Could you check a few things on this model? Use its own coordinates, in mm. Face numbers are marked on the shaded views. A direction names the side the tool comes from. Coordinates: 2 decimals unless noted, no trailing zeros. Order: outer loops, then holes, each group sorted by start corner. A loop starts at its lowest first (then second) coordinate and runs counter-clockwise, first axis right, second up. Notation, with made-up numbers: (22.5, 34.25) - (55.5, 34.25) arc R20 ccw to (55.5, 40.25) - close; hole circle Ø5 at (2, 56.25). An arc over 180 degrees is marked (long way). Answer as CSV lines item,"result". Start each with the question number.
1. I want a section at A-A, the plane z = 7. List the corners of the cut face in (x, y) for me.
2. Thinking about a two-plate mould opening in Y: for the marked faces 4, 5 and 6, which applies, released by +Y, released by -Y, zero draft, split by the parting line, or undercut?
3. For the marked faces 1, 2 and 3, which set-ups out of +Z, -Z, +X, -X, +Y, -Y let a thin tool reach every point of the face, with its end or its side?
4. I want a section at B-B, the plane y = 0. List the corners of the cut face in (x, z) for me (3 decimals).
5. For pin 1 (4 mm diameter, centred on x = 0.43, y = 0, fed in from -Z); pin 2 (3 mm diameter, centred on x = 0.5, y = -2.5, fed in from +Z) (3 decimals), each with a flat end and sliding along its axis, tell me the tip position at first contact or that it passes through.
6. I want a section at C-C, the plane x = 1.25. List the corners of the cut face in (y, z) for me (3 decimals), and give its area (3 significant figures).
7. I need wall thicknesses on probe 1 along Y at (x, z) = (0.5, 3.75); probe 2 along Y at (x, z) = (5.5, 4.25); probe 3 along X at (y, z) = (-1.25, 3). Which ranges of each line are inside material? Lowest first, please.
8. I want a section at D-D, the plane y = -3. List the corners of the cut face in (x, z) for me (3 decimals).
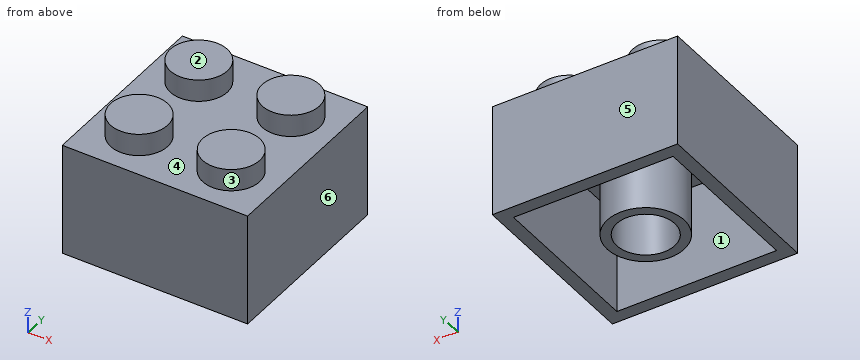
from build123d import *

# Parameters (mm, degrees)
F0_W     = 15.748
F0_H     = 15.748
F1_DEPTH = 9.525
F2_R     = 2.4257
F3_DEPTH = 1.8796
F4_W     = 13.5636
F4_H     = 13.5636
F5_DEPTH = 8.4328
F6_R     = 3.267
F7_DEPTH = 8.4328
F8_R     = 2.467
F9_DEPTH = 8.4328


with BuildPart() as f1:
    # F0 (on Top) → F1 (new body)
    with BuildSketch(Plane.XY):
        with Locations((0.432258, 0.097535)):
            Rectangle(F0_W, F0_H)
    extrude(amount=F1_DEPTH)

    # F2 (on face) → F3 (join)
    with BuildSketch(Plane.XY.offset(9.525)):
        with Locations((-3.479342, 4.009135)):
            Circle(F2_R)
        with Locations((4.343858, 4.009135)):
            Circle(F2_R)
        with Locations((-3.479342, -3.814065)):
            Circle(F2_R)
        with Locations((4.343858, -3.814065)):
            Circle(F2_R)
    extrude(amount=F3_DEPTH)

    # F4 (on face) → F5 (cut)
    with BuildSketch(Plane(origin=(0, 0, 0), x_dir=(1, 0, 0), z_dir=(0, 0, -1))):
        with Locations((0.432258, -0.097535)):
            Rectangle(F4_W, F4_H)
    extrude(amount=-F5_DEPTH, mode=Mode.SUBTRACT)

    # F6 (on face) → F7 (join)
    with BuildSketch(Plane(origin=(0, 0, 8.4328), x_dir=(1, 0, 0), z_dir=(0, 0, -1))):
        with Locations((0.431654, 0)):
            Circle(F6_R)
    extrude(amount=F7_DEPTH)

    # F8 (on face) → F9 (cut)
    with BuildSketch(Plane(origin=(0, 0, 0), x_dir=(1, 0, 0), z_dir=(0, 0, -1))):
        with Locations((0.431654, 0)):
            Circle(F8_R)
    extrude(amount=-F9_DEPTH, mode=Mode.SUBTRACT)


solid = f1.part
Solved:
1,outline,"(-7.44, -7.78) - (8.31, -7.78) - (8.31, 7.97) - (-7.44, 7.97) - close; circle Ø6.53 at (0.43, 0); hole (-6.35, -6.68) - (7.21, -6.68) - (7.21, 6.88) - (-6.35, 6.88) - close; hole circle Ø4.93 at (0.43, 0)"
2,face 4,"undercut"
2,face 5,"released by +Y"
2,face 6,"zero draft"
3,face 1,"-Z"
3,face 2,"+Z, +X, -X, +Y, -Y"
3,face 3,"+Z"
4,outline,"(-7.442, 0) - (-6.35, 0) - (-6.35, 8.433) - (-2.835, 8.433) - (-2.835, 0) - (-2.035, 0) - (-2.035, 8.433) - (2.899, 8.433) - (2.899, 0) - (3.699, 0) - (3.699, 8.433) - (7.214, 8.433) - (7.214, 0) - (8.306, 0) - (8.306, 9.525) - (-7.442, 9.525) - close"
5,pin 1,"stops at z = 8.43"
5,pin 2,"stops at z = 9.525"
6,outline,"(-7.776, 0) - (-6.684, 0) - (-6.684, 8.433) - (-3.163, 8.433) - (-3.163, 0) - (-2.327, 0) - (-2.327, 8.433) - (2.327, 8.433) - (2.327, 0) - (3.163, 0) - (3.163, 8.433) - (6.879, 8.433) - (6.879, 0) - (7.972, 0) - (7.972, 9.525) - (-7.776, 9.525) - close"
6,area,"49.7 mm2"
7,probe 1,"y = -7.78 to -6.68, -3.27 to -2.47, 2.47 to 3.27, 6.88 to 7.97"
7,probe 2,"y = -7.78 to -6.68, 6.88 to 7.97"
7,probe 3,"x = -7.44 to -6.35, -2.59 to -1.7, 2.56 to 3.45, 7.21 to 8.31"
8,outline,"(-7.442, 0) - (-6.35, 0) - (-6.35, 8.433) - (-0.862, 8.433) - (-0.862, 0) - (1.725, 0) - (1.725, 8.433) - (7.214, 8.433) - (7.214, 0) - (8.306, 0) - (8.306, 9.525) - (6.629, 9.525) - (6.629, 11.405) - (2.059, 11.405) - (2.059, 9.525) - (-1.194, 9.525) - (-1.194, 11.405) - (-5.764, 11.405) - (-5.764, 9.525) - (-7.442, 9.525) - close"
